The listing builds one solid part. Answer for the finished solid, in the listing's coordinates (mm). Face numbers are marked on the shaded views. A direction names the side the tool comes from. Round coordinates to 2 decimals unless told otherwise and drop trailing zeros. Write each loop counter-clockwise with the first axis right and the second up, starting at its lowest first coordinate (ties: lowest second). Pieces come first, ordered by that corner, then holes. Notation, with made-up numbers: (15.25, -22) - (24.25, -22) arc R8 ccw to (24.25, -14) - close; hole circle Ø8 at (82.25, 54.5). An arc over 180 degrees is marked (long way). Return JSON: item names as keys, results as strings. Group by question number.
(1) Section D-D, the plane y = 1.75 is taken. Write down the section's boundary in (x, z), then the cut area to 3 significant figures.
(2) Section B-B, the plane z = -1.5 is taken. Write down the section's boundary in (x, y).
(3) Section A-A, the plane y = 0.5 is taken. Write down the section's boundary in (x, z).
(4) Which of the six approach directions +Z, -Z, +X, -X, +Y, -Y give full straight-line access (tool end or side, diameter ignored) to the marked faces 1, 2, 3 and 4?
(5) Each of these flat-tipped pins is pushed along its axis until it touches: pin 1 (1.5 mm diameter, centred on y = 1.5, z = 1, fed in from -X); pin 2 (1.7 mm diameter, centred on x = -8.5, y = 2.5, fed in from +Z); pin 3 (3 mm diameter, centred on y = 6.5, z = -3.5, fed in from -X). Where does it stop, or does it pass through?
(6) Determine the mould class of the marked faces 5, 6, 7 and 8 for opening direction X: +X half, -X half, draft (parallel to the pull), parting line (faces both ways), or undercut.
(7) Find the intervals of material crossed by line 1 along X through (y, z) = (3.75, 4); line 2 along Y through (x, z) = (-8.5, -3.5); line 3 along X through (y, z) = (8.75, 0.5), in increasing order. Write a range as [from, to].
(8) Section C-C, the plane x = 8.5 is taken. Write down the section's boundary in (y, z), then the cut area to 3 significant figures.
```python
from build123d import *

# Parameters (mm, degrees)
BOSS_EXTRUDE1_DEPTH = 5
CUT_EXTRUDE1_REACH  = 18.405
CUT_EXTRUDE2_DEPTH  = 1.8
FILLET1_START       = -5
FILLET1_DEPTH       = 10
FILLET1_2_DEPTH     = 1.969466537
FILLET1_START_2     = 1.530533463
FILLET1_3_DEPTH     = 1.969466537
FILLET1_START_3     = 3.3
FILLET1_4_DEPTH     = 3.7
FILLET2_R           = 1.5
CUT_EXTRUDE3_DEPTH  = 3
CUT_EXTRUDE4_REACH  = 20.279
SKETCH5_W           = 15
SKETCH5_H           = 4.561067126


with BuildPart() as part:
    # Sketch1 → Boss-Extrude1 (new, symmetric)
    with BuildSketch(Plane.XY):
        Polygon((-7.5, 11.5), (7.5, 11.5), (7.5, 3.3), (13.3, 3.3), (13.3, 0), (6, 0), (6, 10), (-6, 10), (-6, 0), (-13.3, 0), (-13.3, 3.3), (-7.5, 3.3), align=None)
    extrude(amount=BOSS_EXTRUDE1_DEPTH, both=True)

    # Sketch2 → Cut-Extrude1 (cut, up to next)
    with BuildSketch(Plane(origin=(0, 3.3, 0), x_dir=(1, 0, 0), z_dir=(0, 1, 0)), mode=Mode.PRIVATE) as cut_extrude1_sk1:
        with BuildLine():
            ThreePointArc((-9.05, -3.5), (-12.05520382, -2.25520382), (-13.3, 0.75))
            Line((-13.3, 0.75), (-13.3, -5))
            Line((-13.3, -5), (-7.5, -5))
            Line((-7.5, -5), (-7.5, -3.5))
            Line((-7.5, -3.5), (-9.05, -3.5))
        make_face()
    cut_extrude1_tool1 = extrude(cut_extrude1_sk1.sketch, amount=-CUT_EXTRUDE1_REACH, mode=Mode.PRIVATE) & part.part
    # Sketch2 → Cut-Extrude1 (cut, up to next)
    with BuildSketch(Plane(origin=(0, 3.3, 0), x_dir=(1, 0, 0), z_dir=(0, 1, 0)), mode=Mode.PRIVATE) as cut_extrude1_sk2:
        with BuildLine():
            ThreePointArc((-13.3, 0.75), (-12.05520382, 3.75520382), (-9.05, 5))
            Line((-9.05, 5), (-13.3, 5))
            Line((-13.3, 5), (-13.3, 0.75))
        make_face()
    cut_extrude1_tool2 = extrude(cut_extrude1_sk2.sketch, amount=-CUT_EXTRUDE1_REACH, mode=Mode.PRIVATE) & part.part
    # Sketch2 → Cut-Extrude1 (cut, up to next)
    with BuildSketch(Plane(origin=(0, 3.3, 0), x_dir=(1, 0, 0), z_dir=(0, 1, 0)), mode=Mode.PRIVATE) as cut_extrude1_sk3:
        with BuildLine():
            ThreePointArc((9.05, 5), (12.05520382, 3.75520382), (13.3, 0.75))
            Line((13.3, 0.75), (13.3, 5))
            Line((13.3, 5), (9.05, 5))
        make_face()
    cut_extrude1_tool3 = extrude(cut_extrude1_sk3.sketch, amount=-CUT_EXTRUDE1_REACH, mode=Mode.PRIVATE) & part.part
    # Sketch2 → Cut-Extrude1 (cut, up to next)
    with BuildSketch(Plane(origin=(0, 3.3, 0), x_dir=(1, 0, 0), z_dir=(0, 1, 0)), mode=Mode.PRIVATE) as cut_extrude1_sk4:
        with BuildLine():
            ThreePointArc((13.3, 0.75), (12.05520382, -2.25520382), (9.05, -3.5))
            Line((9.05, -3.5), (7.5, -3.5))
            Line((7.5, -3.5), (7.5, -5))
            Line((7.5, -5), (13.3, -5))
            Line((13.3, -5), (13.3, 0.75))
        make_face()
    cut_extrude1_tool4 = extrude(cut_extrude1_sk4.sketch, amount=-CUT_EXTRUDE1_REACH, mode=Mode.PRIVATE) & part.part
    add(cut_extrude1_tool1.solids().sort_by_distance((-11.00124, 3.3, 3.726238))[0], mode=Mode.SUBTRACT)
    add(cut_extrude1_tool2.solids().sort_by_distance((-12.350686, 3.3, -4.050686))[0], mode=Mode.SUBTRACT)
    add(cut_extrude1_tool3.solids().sort_by_distance((12.350686, 3.3, -4.050686))[0], mode=Mode.SUBTRACT)
    add(cut_extrude1_tool4.solids().sort_by_distance((11.00124, 3.3, 3.726238))[0], mode=Mode.SUBTRACT)

    # Sketch3 → Cut-Extrude2 (cut)
    with BuildSketch(Plane(origin=(0, 3.3, 0), x_dir=(1, 0, 0), z_dir=(0, 1, 0))):
        Polygon((-9.05, 3.925426481), (-11.8, 2.33771324), (-11.8, -0.83771324), (-9.05, -2.425426481), (-6.3, -0.83771324), (-6.3, 2.33771324), align=None)
        Polygon((9.05, 3.925426481), (6.3, 2.33771324), (6.3, -0.83771324), (9.05, -2.425426481), (11.8, -0.83771324), (11.8, 2.33771324), align=None)
    extrude(amount=-CUT_EXTRUDE2_DEPTH, mode=Mode.SUBTRACT)

    # Fillet1: read off the stored shape, not the designer's step
    # Fillet1 outline → Fillet1 (add)
    with BuildSketch(Plane.XY.offset(FILLET1_START)):
        with BuildLine():
            ThreePointArc((-6, 7), (-5.121320344, 9.121320344), (-3, 10))
            Line((-3, 10), (-6, 10))
            Line((-6, 10), (-6, 7))
        make_face()
        with BuildLine():
            ThreePointArc((3, 10), (5.121320344, 9.121320344), (6, 7))
            Line((6, 7), (6, 10))
            Line((6, 10), (3, 10))
        make_face()
    extrude(amount=FILLET1_DEPTH)

    # Fillet1 2 outline → Fillet1 2 (add)
    with BuildSketch(Plane.XY.offset(FILLET1_START)):
        with BuildLine():
            ThreePointArc((-7.5, 6.3), (-8.378679656, 4.178679656), (-10.5, 3.3))
            Line((-10.5, 3.3), (-7.5, 3.3))
            Line((-7.5, 3.3), (-7.5, 6.3))
        make_face()
        with BuildLine():
            ThreePointArc((10.5, 3.3), (8.378679656, 4.178679656), (7.5, 6.3))
            Line((7.5, 6.3), (7.5, 3.3))
            Line((7.5, 3.3), (10.5, 3.3))
        make_face()
    extrude(amount=FILLET1_2_DEPTH)

    # Fillet1 3 outline → Fillet1 3 (add)
    with BuildSketch(Plane.XY.offset(FILLET1_START_2)):
        with BuildLine():
            ThreePointArc((-7.5, 6.3), (-8.378679656, 4.178679656), (-10.5, 3.3))
            Line((-10.5, 3.3), (-7.5, 3.3))
            Line((-7.5, 3.3), (-7.5, 6.3))
        make_face()
        with BuildLine():
            ThreePointArc((10.5, 3.3), (8.378679656, 4.178679656), (7.5, 6.3))
            Line((7.5, 6.3), (7.5, 3.3))
            Line((7.5, 3.3), (10.5, 3.3))
        make_face()
    extrude(amount=FILLET1_3_DEPTH)

    # Fillet1 4 outline → Fillet1 4 (cut)
    with BuildSketch(Plane(origin=(0, 0, 0), x_dir=(1, 0, 0), z_dir=(0, 1, 0)).offset(FILLET1_START_3)):
        with BuildLine():
            ThreePointArc((10.5, -3.244996871), (9.786126109, -3.435763772), (9.05, -3.5))
            Line((9.05, -3.5), (10.5, -3.5))
            Line((10.5, -3.5), (10.5, -3.244996871))
        make_face()
        Polygon((9.05, 3.925426481), (7.5, 3.030533563), (10.5, 3.030533463), (10.5, 3.08826859), align=None)
        Polygon((10.5, -1.530533463), (7.5, -1.530533463), (9.05, -2.425426481), (10.5, -1.58826859), align=None)
        with BuildLine():
            Line((10.5, 5), (9.05, 5))
            ThreePointArc((9.05, 5), (9.786126109, 4.935763772), (10.5, 4.744996871))
            Line((10.5, 4.744996871), (10.5, 5))
        make_face()
        with BuildLine():
            ThreePointArc((-9.05, -3.5), (-9.786126109, -3.435763772), (-10.5, -3.244996871))
            Line((-10.5, -3.244996871), (-10.5, -3.5))
            Line((-10.5, -3.5), (-9.05, -3.5))
        make_face()
        Polygon((-9.05, 3.925426481), (-10.5, 3.08826859), (-10.5, 3.030533463), (-7.5, 3.030533463), align=None)
        Polygon((-7.5, -1.530533463), (-10.5, -1.530533463), (-10.5, -1.58826859), (-9.05, -2.425426481), align=None)
        with BuildLine():
            Line((-9.05, 5), (-10.5, 5))
            Line((-10.5, 5), (-10.5, 4.744996871))
            ThreePointArc((-10.5, 4.744996871), (-9.786126109, 4.935763772), (-9.05, 5))
        make_face()
    extrude(amount=FILLET1_4_DEPTH, mode=Mode.SUBTRACT)

    # Fillet2
    fillet2_edges = [part.edges().sort_by_distance(p)[0] for p in [
        (-7.5, 11.5, 0),
        (7.5, 11.5, 0),
    ]]
    fillet(fillet2_edges, radius=FILLET2_R)

    # Sketch4 → Cut-Extrude3 (cut)
    with BuildSketch(Plane(origin=(0, 0, 0), x_dir=(1, 0, 0), z_dir=(0, 1, 0))):
        with BuildLine():
            Line((-9.05, -0.75), (9.05, -0.75))
            ThreePointArc((9.05, -0.75), (10.55, 0.75), (9.05, 2.25))
            Line((9.05, 2.25), (-9.05, 2.25))
            ThreePointArc((-9.05, 2.25), (-10.55, 0.75), (-9.05, -0.75))
        make_face()
    extrude(amount=CUT_EXTRUDE3_DEPTH, mode=Mode.SUBTRACT)

    # Cut-Extrude4: up to this face of the body (flat: up to its plane)
    cut_extrude4_end = Plane(part.part.faces().sort_by_distance((6.935820896, 3.3, -0.75))[0])
    # Sketch5 → Cut-Extrude4 (cut, up to the picked face)
    with BuildSketch(Plane(origin=(0, 0, 0), x_dir=(1, 0, 0), z_dir=(0, 1, 0)), mode=Mode.PRIVATE) as cut_extrude4_sk1:
        with Locations((0, 0.75)):
            Rectangle(SKETCH5_W, SKETCH5_H)
    cut_extrude4_tool1 = split(extrude(cut_extrude4_sk1.sketch, amount=CUT_EXTRUDE4_REACH, mode=Mode.PRIVATE), bisect_by=cut_extrude4_end, keep=Keep.BOTH, mode=Mode.PRIVATE)
    add(cut_extrude4_tool1.solids().sort_by(Axis((0, 0, -0.75), (0, 1, 0)))[0], mode=Mode.SUBTRACT)


solid = part.part
```
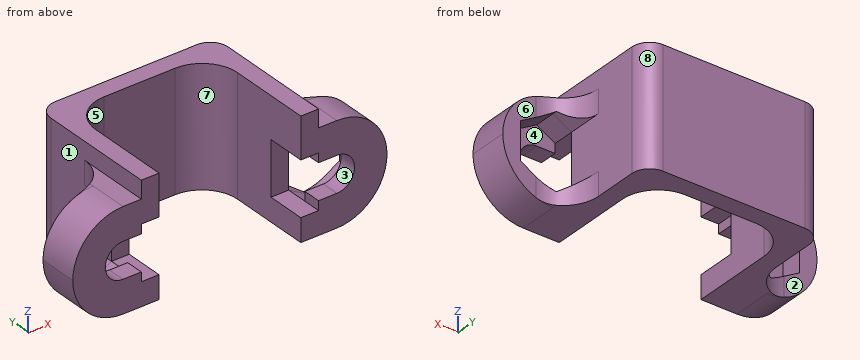
Working result:
{
 "1": {"outline": "(-11.8, -2.34) - (-11.8, 0.84) - (-9.05, 2.43) - (-7.5, 1.53) - (-6, 1.53) - (-6, 5) - (-7.5, 5) - (-7.5, 3.5) - (-9.05, 3.5) arc R4.25 ccw to (-9.05, -5) - (-6, -5) - (-6, -3.03) - (-7.5, -3.03) - (-9.05, -3.93) - close; (6, -5) - (9.05, -5) arc R4.25 ccw to (9.05, 3.5) - (7.5, 3.5) - (7.5, 5) - (6, 5) - (6, 1.53) - (7.5, 1.53) - (9.05, 2.43) - (11.8, 0.84) - (11.8, -2.34) - (9.05, -3.93) - (7.5, -3.03) - (6, -3.03) - close", "area": "56.3 mm^2"},
 "2": {"outline": "(-13.23, 0) - (-10.35, 0) - (-10.35, 1.5) - (-11.8, 1.5) - (-11.8, 3.3) - (-13.23, 3.3) - close; (-7.5, 3.3) - (-6, 3.3) - (-6, 7) arc R3 cw to (-3, 10) - (3, 10) arc R3 cw to (6, 7) - (6, 3.3) - (7.5, 3.3) - (7.5, 10) arc R1.5 ccw to (6, 11.5) - (-6, 11.5) arc R1.5 ccw to (-7.5, 10) - close; (10.35, 0) - (13.23, 0) - (13.23, 3.3) - (11.8, 3.3) - (11.8, 1.5) - (10.35, 1.5) - close"},
 "3": {"outline": "(-9.05, -5) - (-6, -5) - (-6, -3.03) - (-7.5, -3.03) - (-7.5, -2.25) - (-9.05, -2.25) arc R1.5 cw to (-9.05, 0.75) - (-7.5, 0.75) - (-7.5, 1.53) - (-6, 1.53) - (-6, 5) - (-7.5, 5) - (-7.5, 3.5) - (-9.05, 3.5) arc R4.25 ccw to start; (6, -5) - (9.05, -5) arc R4.25 ccw to (9.05, 3.5) - (7.5, 3.5) - (7.5, 5) - (6, 5) - (6, 1.53) - (7.5, 1.53) - (7.5, 0.75) - (9.05, 0.75) arc R1.5 cw to (9.05, -2.25) - (7.5, -2.25) - (7.5, -3.03) - (6, -3.03) - close"},
 "4": {"face 1": "-X, +Y", "face 2": "+Z, -Z, -X, +Y", "face 3": "+Y, -Y", "face 4": "+Y"},
 "5": {"pin 1": "stops at x = -13.18", "pin 2": "stops at z = 3.5", "pin 3": "stops at x = -7.8"},
 "6": {"face 5": "undercut", "face 6": "draft", "face 7": "undercut", "face 8": "+X half"},
 "7": {"line 1": "x = [-7.5, -6], [6, 7.5]", "line 2": "y = [0, 1.5]", "line 3": "x = [-7.5, -5.44], [5.44, 7.5]"},
 "8": {"outline": "(0, -5) - (4.06, -5) - (4.06, -3.61) - (1.5, -3.61) - (1.5, -2.25) - (0, -2.25) - close; (0, 0.75) - (1.5, 0.75) - (1.5, 2.11) - (4.06, 2.11) - (4.06, 3.5) - (0, 3.5) - close", "area": "15.4 mm^2"}
}
